```python
from build123d import *

# Parameters (mm, degrees)
CUT_EXTRUDE1_DEPTH      = 66.991135768
CUT_EXTRUDE1_DEPTH_BACK = 66.991135768
CUT_REVOLVE1_ANGLE      = 45
CIRPATTERN1_COUNT       = 4


with BuildPart() as part:
    # Sketch1 → Revolve1 (revolve)
    with BuildSketch(Plane.XY, mode=Mode.PRIVATE) as revolve1_sk:
        Polygon((6.35, 0), (6.35, 38.1), (16.102954744, 38.1), (38.1, 0), align=None)
    revolve(revolve1_sk.sketch.rotate(Axis((0, 0, 0), (0, 1, 0)), 90), axis=Axis((0, 0, 0), (0, 1, 0)))

    # Sketch2 → Cut-Extrude1 (cut, two sides: drawn at the far end of the back side and taken through both)
    with BuildSketch(Plane(origin=(0, 38.1, 0), x_dir=(1, 0, 0), z_dir=(0, 1, 0)).offset(-CUT_EXTRUDE1_DEPTH_BACK)):
        with BuildLine():
            Line((1.524, 7.62), (-1.524, 7.62))
            Line((-1.524, 7.62), (-1.524, 6.164407839))
            ThreePointArc((-1.524, 6.164407839), (0, 6.35), (1.524, 6.164407839))
            Line((1.524, 6.164407839), (1.524, 7.62))
        make_face()
    extrude(amount=CUT_EXTRUDE1_DEPTH + CUT_EXTRUDE1_DEPTH_BACK, mode=Mode.SUBTRACT)

    # Sketch3 → Cut-Revolve1 (revolve, symmetric, cut)
    with BuildSketch(Plane(origin=(0, 0, 0), x_dir=(0, 0, -1), z_dir=(1, 0, 0))) as cut_revolve1_sk:
        Polygon((16.102954744, 38.1), (14.832954744, 38.1), (36.83, 0), (38.1, 0), align=None)
    cut_revolve1 = revolve(axis=Axis((0, 0, 0), (0, 1, 0)), revolution_arc=CUT_REVOLVE1_ANGLE / 2, mode=Mode.SUBTRACT)
    cut_revolve1 = cut_revolve1 + revolve(cut_revolve1_sk.sketch, axis=Axis((0, 0, 0), (0, -1, 0)), revolution_arc=CUT_REVOLVE1_ANGLE / 2, mode=Mode.SUBTRACT)

    # CirPattern1: Cut-Revolve1 ×4 about axis
    cirpattern1_axis = Axis((0, 38.1, 0), (0, -1, 0))
    for i in range(1, CIRPATTERN1_COUNT):
        add(cut_revolve1.rotate(cirpattern1_axis, i * 360 / CIRPATTERN1_COUNT), mode=Mode.SUBTRACT)


solid = part.part
```
The model under review builds one solid part; all positions refer to its coordinate system, in mm. A direction names the side the tool comes from. Round coordinates to 2 decimals unless told otherwise and drop trailing zeros. Order: outer loops, then holes, each group sorted by start corner. A loop starts at its lowest first (then second) coordinate and runs counter-clockwise, first axis right, second up.
(1) Tool access review of faces 1 (the face through (10.108, 19.139, -24.402)), 2 (the face through (-10.108, 19.139, 24.402)), 3 (the face through (24.402, 19.139, 10.108)), 4 (the face through (-24.402, 19.139, -10.108)): name each direction out of +Z, -Z, +X, -X, +Y, -Y from which nothing blocks a thin tool from reaching the whole face with its end or side.
Working result:
face 1: -Z, +Y
face 2: +Z, +Y
face 3: +X, +Y
face 4: -X, +Y
(2) Take a section at D-D, the plane y = 24. State the section outline as (x, z) points, plus the area to 3 significant figures.
Working result:
outline: (-22.4, -9.28) arc R24.24 ccw to (-9.28, -22.4) - (-8.79, -21.22) arc R22.97 ccw to (8.79, -21.22) - (9.28, -22.4) arc R24.24 ccw to (22.4, -9.28) - (21.22, -8.79) arc R22.97 ccw to (21.22, 8.79) - (22.4, 9.28) arc R24.24 ccw to (9.28, 22.4) - (8.79, 21.22) arc R22.97 ccw to (-8.79, 21.22) - (-9.28, 22.4) arc R24.24 ccw to (-22.4, 9.28) - (-21.22, 8.79) arc R22.97 ccw to (-21.22, -8.79) - close; hole (-1.52, -7.62) - (1.52, -7.62) - (1.52, -6.16) arc R6.35 ccw (long way) to (-1.52, -6.16) - close
area: 1,620 mm2
(3) Take a section at B-B, the plane z = 0. State the section outline as (x, y) points.
Working result:
outline: (-36.83, 0) - (-6.35, 0) - (-6.35, 38.1) - (-14.83, 38.1) - close; (6.35, 0) - (36.83, 0) - (14.83, 38.1) - (6.35, 38.1) - close
(4) For P1, Ø6, axis at x = 17.5, y = 33, coming from the +Z side; P2, Ø0.9, axis at x = 0.5, y = 21.5, coming from the +Z side; P3, Ø4, axis at y = 8.5, z = 29, coming from the -X side, all flat-tipped, find the tip position at first contact; note any pin that passes through.
Working result:
P1: stops at z = 13.25
P2: stops at z = 24.67
P3: stops at x = -19.94
(5) Wall thickness on L1, parallel to X at y = 13, z = 5.5; L2, parallel to Y at x = 23, z = -2.5; L3, parallel to Z at x = 19.5, y = 20: over which ranges is each line inside the solid? List them lowest first.
Working result:
L1: x = -28.8 to -3.17, 3.17 to 28.8
L2: y = 0 to 23.72
L3: z = -18.02 to 18.02
(6) Take a section at A-A, the plane x = 0. State the section outline as (y, z) points, plus the area to 3 significant figures.
Working result:
outline: (0, -36.83) - (38.1, -14.83) - (38.1, -7.62) - (0, -7.62) - close; (0, 6.35) - (38.1, 6.35) - (38.1, 14.83) - (0, 36.83) - close
area: 1,440 mm2
(7) Mouldability with a two-part tool opening along Z and no side actions: class faces 5 (the face through (19.17, 18.78, 19.38)), 6 (the face through (-0.258, 19.317, 6.345)), 7 (the face through (19.38, 18.78, -19.17)) as released by +Z, released by -Z, zero draft, split by the parting line, or undercut.
Working result:
face 5: released by +Z
face 6: undercut
face 7: released by -Z
(8) Take a section at C-C, the plane y = 19. State the section outline as (x, z) points, plus the area to 3 significant figures.
Working result:
outline: (-25.07, -10.38) arc R27.13 ccw to (-10.38, -25.07) - (-9.9, -23.89) arc R25.86 ccw to (9.9, -23.89) - (10.38, -25.07) arc R27.13 ccw to (25.07, -10.38) - (23.89, -9.9) arc R25.86 ccw to (23.89, 9.9) - (25.07, 10.38) arc R27.13 ccw to (10.38, 25.07) - (9.9, 23.89) arc R25.86 ccw to (-9.9, 23.89) - (-10.38, 25.07) arc R27.13 ccw to (-25.07, 10.38) - (-23.89, 9.9) arc R25.86 ccw to (-23.89, -9.9) - close; hole (-1.52, -7.62) - (1.52, -7.62) - (1.52, -6.16) arc R6.35 ccw (long way) to (-1.52, -6.16) - close
area: 2,080 mm2
